from build123d import *

# Parameters (mm, degrees)
FEATURE_B_DEPTH     = 7.706067936
FEATURE_START       = 25.4
SKETCH3_R           = 11.162804955
FEATURE_A_DEPTH     = 25.4
SKETCH5_W           = 65.757777778
SKETCH5_H           = 7.184204897
FEATURE_C_DEPTH     = 25.4
SKETCH6_W           = 25.4
SKETCH6_H           = 1.128888889
FEATURE_D_DEPTH     = 38.1
SKETCH8_W           = 25.4
SKETCH8_H           = 26.528888889
BOSS_EXTRUDE5_DEPTH = 22.354838115


with BuildPart() as part:
    # Sketch1 → Feature B (new body)
    with BuildSketch(Plane.YZ):
        with BuildLine():
            Line((0, 0), (0, 25.4))
            Line((0, 25.4), (22.32560991, 25.4))
            Line((22.32560991, 25.4), (22.32560991, 0))
            ThreePointArc((22.32560991, 0), (11.162804955, -11.162804955), (0, 0))
        make_face()
    extrude(amount=FEATURE_B_DEPTH)

    # Sketch3 → Feature A (add)
    with BuildSketch(Plane(origin=(0, 0, 0), x_dir=(0, -1, 0), z_dir=(-1, 0, 0)).offset(FEATURE_START)):
        with Locations(Location((-11.162804955, 0, 0), (0, 0, 90))):
            Circle(SKETCH3_R)
    extrude(amount=-FEATURE_A_DEPTH)

    # Sketch5 → Feature C (add)
    with BuildSketch(Plane.YZ.offset(7.706067936)):
        with Locations((11.162804955, 28.992102448)):
            Rectangle(SKETCH5_W, SKETCH5_H)
    extrude(amount=-FEATURE_C_DEPTH)

    # Sketch6 → Feature D (add)
    with BuildSketch(Plane.XY.offset(32.584204897)):
        with Locations((-4.993932064, -21.151639489)):
            Rectangle(SKETCH6_W, SKETCH6_H)
        with Locations((-4.993932064, 43.4772494)):
            Rectangle(SKETCH6_W, SKETCH6_H)
    extrude(amount=FEATURE_D_DEPTH)

    # Sketch8 → Boss-Extrude5 (add)
    with BuildSketch(Plane.XY.offset(70.684204897)):
        with Locations((-4.993932064, -8.451639489)):
            Rectangle(SKETCH8_W, SKETCH8_H)
        with Locations((-4.993932064, 30.7772494)):
            Rectangle(SKETCH8_W, SKETCH8_H)
    extrude(amount=BOSS_EXTRUDE5_DEPTH)


solid = part.part
Work out the finished part from the listing and answer in its coordinate system (mm). A direction names the side the tool comes from. Give positions to 0.01 mm unless a question says otherwise; leave off trailing zeros. Write each loop counter-clockwise with the first axis right and the second up, starting at its lowest first coordinate (ties: lowest second). Pieces come first, ordered by that corner, then holes. Notation, with made-up numbers: (-11.75, 59) - (5.25, 59) arc R23 cw to (5.25, 82) - close; hole circle Ø5 at (89, -36). An arc over 180 degrees is marked (long way). One line per item, written item: value. Start each with the question number.
1. Find section B-B (y = 35.5). Write down the section's boundary in (x, z).
2. Consider probe 1 along Y at (x, z) = (-0.5, 83); probe 2 along Z at (x, y) = (-7, 30); probe 3 along Y at (x, z) = (1, 38). Determine where each line is inside the solid, lowest interval first.
3. Find section D-D (x = 3). Write down the section's boundary in (y, z).
4. Find section C-C (x = -2.5). Write down the section's boundary in (y, z), then the cut area to 3 significant figures.
5. Find section A-A (z = 83). Write down the section's boundary in (x, y), then the cut area to 3 significant figures.
6. For a pull along Y with two mould halves and no side action, classify faces 4 (the flat face through (-5, 42.913, 51)), 5 (the cylindrical face through (-9.079, 11.654, -11.152)), 6 (the flat face through (-5, -8, 93.039)), 7 (the flat face through (-5, 30, 70.684)) as +Y half, -Y half, draft (parallel to the pull), parting line (faces both ways), or undercut.
7. For faces 1 (the flat face through (4, 22.326, 13)), 2 (the flat face through (-5, 17.513, 82)), 3 (the flat face through (-17.694, 3, 74)), determine the directions among +Z, -Z, +X, -X, +Y, -Y from which every point of the face is accessible in a straight line to the end or side of a thin tool.
8. Given pin 1 (2 mm diameter, centred on x = -12, y = 19.5, fed in from -Z); pin 2 (6 mm diameter, centred on x = 2.5, z = 18.5, fed in from -Y); pin 3 (8 mm diameter, centred on y = -10, z = 28, fed in from -X), each flat-ended and moving along its own axis, determine where each tip first touches the part or whether it passes through.
Geometry results:
1. outline: (-17.69, 25.4) - (7.71, 25.4) - (7.71, 32.58) - (-17.69, 32.58) - close; (-17.69, 70.68) - (7.71, 70.68) - (7.71, 93.04) - (-17.69, 93.04) - close
2. probe 1: -21.72 to 4.81, 17.51 to 44.04
2. probe 2: 25.4 to 32.58, 70.68 to 93.04
2. probe 3: -21.72 to -20.59, 42.91 to 44.04
3. outline: (-21.72, 25.4) - (0, 25.4) - (0, 0) arc R11.16 ccw to (22.33, 0) - (22.33, 25.4) - (44.04, 25.4) - (44.04, 93.04) - (17.51, 93.04) - (17.51, 70.68) - (42.91, 70.68) - (42.91, 32.58) - (-20.59, 32.58) - (-20.59, 70.68) - (4.81, 70.68) - (4.81, 93.04) - (-21.72, 93.04) - close
4. outline: (-21.72, 25.4) - (44.04, 25.4) - (44.04, 93.04) - (17.51, 93.04) - (17.51, 70.68) - (42.91, 70.68) - (42.91, 32.58) - (-20.59, 32.58) - (-20.59, 70.68) - (4.81, 70.68) - (4.81, 93.04) - (-21.72, 93.04) - close; circle Ø22.33 at (11.16, 0)
4. area: 2,140 mm2
5. outline: (-17.69, -21.72) - (7.71, -21.72) - (7.71, 4.81) - (-17.69, 4.81) - close; (-17.69, 17.51) - (7.71, 17.51) - (7.71, 44.04) - (-17.69, 44.04) - close
5. area: 1,350 mm2
6. face 4: undercut
6. face 5: parting line
6. face 6: draft
6. face 7: undercut
7. face 1: -Z, +X, -X, +Y
7. face 2: +Z, +X, -X
7. face 3: +Z, -X, +Y, -Y
8. pin 1: z = -8.41
8. pin 2: y = 0
8. pin 3: x = -17.69
